Geometry: see drawing. Coordinates: mm, zero at the bounding-box minimum. Round coordinates to 2 decimals unless told otherwise and drop trailing zeros. Loops run counter-clockwise (first coordinate to the right, second up) from the corner with the lowest first, then second, coordinate; pieces in that order, holes last. Notation, with made-up numbers: (26.5, 39.5) - (79.5, 39.5) arc R25 ccw to (79.5, 75.5) - close; hole circle Ø6 at (55, 25.25). An arc over 180 degrees is marked (long way). Use CSV: the item, a comma, the result in double quotes.
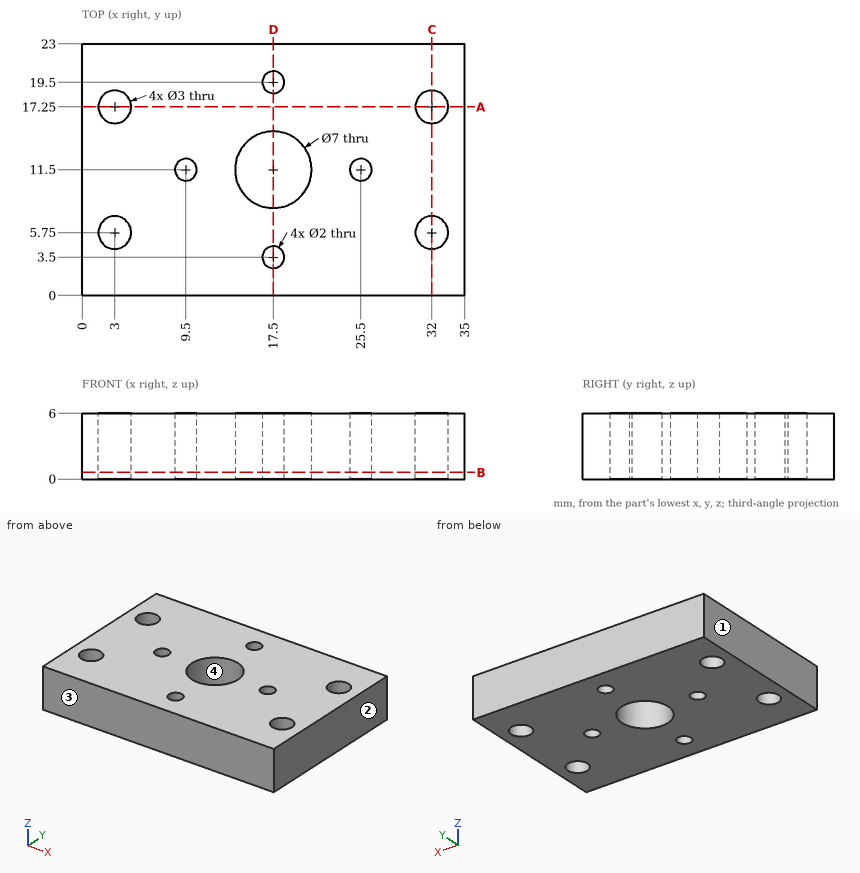
Item 1: Material intervals for line 1 (Y direction, x = 17.5, z = 2.65); line 2 (Y direction, x = 25.5, z = 4.85); line 3 (Y direction, x = 3.5, z = 4.75), sorted ascending.
Final values:
line 1,"y = 0 to 2.5, 4.5 to 8, 15 to 18.5, 20.5 to 23"
line 2,"y = 0 to 10.5, 12.5 to 23"
line 3,"y = 0 to 4.34, 7.16 to 15.84, 18.66 to 23"
Item 2: Section B-B on z = 0.6. Give the number of separate pieces and of enclosed holes in the cut face, plus the area to 3 significant figures.
Final values:
separate pieces,"1"
enclosed holes,"9"
area,"726 mm²"
Item 3: Mould query, pull axis X, two halves, no side actions, for the marked faces 1, 2, 3 and 4. Classes: released by +X, released by -X, zero draft, split by the parting line, or undercut.
Final values:
face 1,"released by -X"
face 2,"released by +X"
face 3,"zero draft"
face 4,"undercut"
Item 4: Section D-D on x = 17.5. Return the cut outline in (y, z), plus the area to 3 significant figures.
Final values:
outline,"(0, 0) - (2.5, 0) - (2.5, 6) - (0, 6) - close; (4.5, 0) - (8, 0) - (8, 6) - (4.5, 6) - close; (15, 0) - (18.5, 0) - (18.5, 6) - (15, 6) - close; (20.5, 0) - (23, 0) - (23, 6) - (20.5, 6) - close"
area,"72.0 mm²"
Item 5: Pin query (flat end, axial travel): P1, Ø1.8, axis at x = 32, y = 17.25, coming from the +Z side; P2, Ø3, axis at x = 17.5, y = 19.5, coming from the -Z side. Return the tip coordinate at first contact, or that it passes through.
Final values:
P1,"passes through"
P2,"stops at z = 0"
Item 6: Section C-C on x = 32. Return the cut outline in (y, z).
Final values:
outline,"(0, 0) - (4.25, 0) - (4.25, 6) - (0, 6) - close; (7.25, 0) - (15.75, 0) - (15.75, 6) - (7.25, 6) - close; (18.75, 0) - (23, 0) - (23, 6) - (18.75, 6) - close"
Item 7: Section A-A on y = 17.25. Return the cut outline in (x, z).
Final values:
outline,"(0, 0) - (1.5, 0) - (1.5, 6) - (0, 6) - close; (4.5, 0) - (30.5, 0) - (30.5, 6) - (4.5, 6) - close; (33.5, 0) - (35, 0) - (35, 6) - (33.5, 6) - close"
